Read the model definition and answer for the solid it produces. Units are mm, in the model's axes. Give positions to 0.01 mm unless a question says otherwise; leave off trailing zeros. Order: outer loops, then holes, each group sorted by start corner. A loop starts at its lowest first (then second) coordinate and runs counter-clockwise, first axis right, second up. Notation, with made-up numbers: (-35, 64) - (-28, 64) arc R20 cw to (-28, 73) - close; hole circle Ø9 at (-23, 0). An arc over 180 degrees is marked (long way). Return JSON: item names as keys, results as strings.
Autodesk Inventor part; units mm, degrees
ref_plane "YZ Plane" through (0, 0, 0) normal (1, 0, 0) x (0, 1, 0)
ref_plane "XZ Plane" through (0, 0, 0) normal (0, 1, 0) x (-1, 0, 0)
ref_plane "XY Plane" through (0, 0, 0) normal (0, 0, 1) x (1, 0, 0)
sketch "Sketch1" plane through (0, 0, 0) normal (0, 1, 0) x (-1, 0, 0)
  circle A0 centre (0, 0) radius 25.4
  dimension "d0" = 50.8
extrude "Extrusion1" add sketch "Sketch1" along normal blind 38.1
sketch "Sketch5" plane through (0, 38.1, 0) normal (0, 1, 0) x (1, 0, 0)
  circle A0 centre (0, 0) radius 22.225
  dimension "d32" = 44.45
extrude "Extrusion4" cut sketch "Sketch5" against normal through all
fillet "Fillet1" radius 0.7937 2 edges at (-22.225, 38.1, 0) (25.4, 38.1, 0)
properties part number "WL-0012" material "Aluminum 6061"
Q1. A cutting plane is placed at B-B (z = 0). Write down the section's boundary in (x, y) (3 decimals).
Values:
{"outline": "(-25.4, 0) - (-22.225, 0) - (-22.225, 37.306) arc R0.794 ccw to (-23.019, 38.1) - (-24.606, 38.1) arc R0.794 ccw to (-25.4, 37.306) - close; (22.225, 0) - (25.4, 0) - (25.4, 37.306) arc R0.794 ccw to (24.606, 38.1) - (23.019, 38.1) arc R0.794 ccw to (22.225, 37.306) - close"}
Q2. Determine the mould class of faces 1 (the cylindrical face through (5.506, 18.392, 24.796)), 2 (the cylindrical face through (21.199, 18.914, -6.676)), 3 (the flat face through (0.1, 0, -22.5)) for opening direction Z: released by +Z, released by -Z, zero draft, split by the parting line, or undercut.
Values:
{"face 1": "split by the parting line", "face 2": "undercut", "face 3": "zero draft"}
Q3. Consider L1, parallel to Z at x = 0, y = 8 (3 decimals); L2, parallel to X at y = 18, z = -8; L3, parallel to Y at x = -14.5, z = -20. Determine where each line is inside the solid, lowest interval first.
Values:
{"L1": "z = -25.4 to -22.225, 22.225 to 25.4", "L2": "x = -24.11 to -20.74, 20.74 to 24.11", "L3": "y = 0 to 38.09"}
Q4. A cutting plane is placed at A-A (x = 0). Write down the section's boundary in (y, z) (3 decimals).
Values:
{"outline": "(0, -25.4) - (37.306, -25.4) arc R0.794 ccw to (38.1, -24.606) - (38.1, -23.019) arc R0.794 ccw to (37.306, -22.225) - (0, -22.225) - close; (0, 22.225) - (37.306, 22.225) arc R0.794 ccw to (38.1, 23.019) - (38.1, 24.606) arc R0.794 ccw to (37.306, 25.4) - (0, 25.4) - close"}
Q5. A cutting plane is placed at C-C (y = 30). Write down the section's boundary in (x, z) (3 decimals).
Values:
{"outline": "circle Ø50.8 at (0, 0); hole circle Ø44.45 at (0, 0)"}
Q6. Given pin 1 (4 mm diameter, centred on y = 19.5, z = -4.5, fed in from +X); pin 2 (1.5 mm diameter, centred on x = 1.5, y = 13.5, fed in from -Z); pin 3 (2 mm diameter, centred on y = 29, z = -17.5, fed in from -X), each flat-ended and moving along its own axis, determine where each tip first touches the part or whether it passes through.
Values:
{"pin 1": "stops at x = 25.28", "pin 2": "stops at z = -25.39", "pin 3": "stops at x = -19.31"}
